Part model, mm, in its own coordinate system. A direction names the side the tool comes from. Round coordinates to 2 decimals unless told otherwise and drop trailing zeros. Write each loop counter-clockwise with the first axis right and the second up, starting at its lowest first coordinate (ties: lowest second). Pieces come first, ordered by that corner, then holes. Notation, with made-up numbers: M 31.5,62 L 67.5,62 A27 ccw 67.5,78 Z; hole C -4,42 d4. An arc over 180 degrees is marked long. Answer as a JSON object with one key per item and string values. Group by question number.
1. Band-saw the part on A-A, the plane x = 3.75. Write the cut outline in (y, z), plus the area to 3 significant figures.
2. Drill centre lines: line 1 (Z direction, x = -0.5, y = 0); line 2 (Y direction, x = 6.75, z = 6.5); line 3 (Y direction, x = 6.75, z = 0). Where is each one in solid material? Low to high. Write a range as from..to.
3. Drop flat-ended pins along their axis: pin 1 (1.5 mm diameter, centred on x = 3, z = 14.5, fed in from -Y); pin 2 (10 mm diameter, centred on y = 12.5, z = 12.5, fed in from +X); pin 3 (0.6 mm diameter, centred on y = 4, z = 4, fed in from +X). Give the stop position or say it passes through.
4. Band-saw the part on B-B, the plane y = 0. Count the separate pieces of the cut face and the enclosed holes in it, plus the area to 3 significant figures.
5. Band-saw the part on C-C, the plane x = 10. Write the cut outline in (y, z), plus the area to 3 significant figures.
6. Band-saw the part on D-D, the plane x = -0.75. Write the cut outline in (y, z).
7. Two-plate mould, pull along Z, no slides. Class faces 1 (the face through (-2.63, 13.926, 4.385)), 2 (the face through (4.105, 17.717, 5.579)), 3 (the face through (18.591, -4, 4)): +Z half, -Z half, draft (parallel to the pull), parting line (faces both ways), or undercut.
8. Which spindle directions (+Z, -Z, +X, -X, +Y, -Y) get a long thin tool onto all of the face, cutting with end or side? Do faces 4 (the face through (18.591, 0, -5)), 5 (the face through (18.084, 4.605, 3.225)), 6 (the face through (18.591, -5, 0)), 7 (the face through (18.591, 5, 0)). Say none if no direction does.
from build123d import *

# Parameters (mm, degrees)
SKETCH2_R           = 1.35
CUT_EXTRUDE1_DEPTH  = 10
SKETCH3_R           = 3.977137015
SKETCH3_R_2         = 1
BOSS_EXTRUDE1_DEPTH = 2
FILLET1_R           = 1
SKETCH4_R           = 1
CUT_EXTRUDE2_DEPTH  = 1


with BuildPart() as part:
    # Sketch1 → Revolve1 (revolve)
    with BuildSketch(Plane.XY):
        Polygon((-9.308622786, 16.6), (3.091377214, 16.6), (3.091377214, 18.57463979), (5.091377214, 18.57463979), (5.091377214, 18.07463979), (4.591377214, 18.07463979), (4.591377214, 17.07463979), (7.591377214, 14.07463979), (7.591377214, 6.75), (17.591377214, 6.75), (17.591377214, 0), (6.591377214, 0), (5.591377214, 0), (5.591377214, 13.246212665), (4.237589879, 14.6), (-9.308622786, 14.6), align=None)
    revolve(axis=Axis((-25, 0, 0), (1, 0, 0)))

    # Sketch2 → Cut-Extrude1 (cut)
    with BuildSketch(Plane.ZY.offset(-5.591377214)):
        with Locations((0, 9.5)):
            Circle(SKETCH2_R)
        with Locations((6.717514421, 6.717514421)):
            Circle(SKETCH2_R)
        with Locations((9.5, 0)):
            Circle(SKETCH2_R)
        with Locations((6.717514421, -6.717514421)):
            Circle(SKETCH2_R)
        with Locations((0, -9.5)):
            Circle(SKETCH2_R)
        with Locations((-6.717514421, -6.717514421)):
            Circle(SKETCH2_R)
        with Locations((-9.5, 0)):
            Circle(SKETCH2_R)
        with Locations((-6.717514421, 6.717514421)):
            Circle(SKETCH2_R)
    extrude(amount=-CUT_EXTRUDE1_DEPTH, mode=Mode.SUBTRACT)

    # Sketch3 → Boss-Extrude1 (add)
    with BuildSketch(Plane(origin=(17.591377214, 0, 0), x_dir=(0, 0, -1), z_dir=(1, 0, 0))):
        Circle(SKETCH3_R)
        with Locations((0, 5.320667936)):
            Circle(SKETCH3_R_2)
        with Locations((3.762280378, 3.762280378)):
            Circle(SKETCH3_R_2)
        with Locations((5.320667936, 0)):
            Circle(SKETCH3_R_2)
        with Locations((3.762280378, -3.762280378)):
            Circle(SKETCH3_R_2)
        with Locations((0, -5.320667936)):
            Circle(SKETCH3_R_2)
        with Locations((-3.762280378, -3.762280378)):
            Circle(SKETCH3_R_2)
        with Locations((-5.320667936, 0)):
            Circle(SKETCH3_R_2)
        with Locations((-3.762280378, 3.762280378)):
            Circle(SKETCH3_R_2)
    extrude(amount=BOSS_EXTRUDE1_DEPTH)

    # Fillet1
    fillet1_edges = [part.edges().sort_by_distance(p)[0] for p in [
        (19.591377214, 0, 3.977137015),
    ]]
    fillet(fillet1_edges, radius=FILLET1_R)

    # Sketch4 → Cut-Extrude2 (cut)
    with BuildSketch(Plane(origin=(19.591377214, 0, 0), x_dir=(0, 0, -1), z_dir=(1, 0, 0))):
        with Locations((0, 5.320667936)):
            Circle(SKETCH4_R)
        with Locations((3.762280378, 3.762280378)):
            Circle(SKETCH4_R)
        with Locations((5.320667936, 0)):
            Circle(SKETCH4_R)
        with Locations((3.762280378, -3.762280378)):
            Circle(SKETCH4_R)
        with Locations((0, -5.320667936)):
            Circle(SKETCH4_R)
        with Locations((-3.762280378, -3.762280378)):
            Circle(SKETCH4_R)
        with Locations((-5.320667936, 0)):
            Circle(SKETCH4_R)
        with Locations((-3.762280378, 3.762280378)):
            Circle(SKETCH4_R)
    extrude(amount=-CUT_EXTRUDE2_DEPTH, mode=Mode.SUBTRACT)


solid = part.part
Worked answers:
{
 "1": {"outline": "C 0,0 d37.15; hole C 0,0 d29.2", "area": "414 mm^2"},
 "2": {"line 1": "z = -16.6..-14.6, 14.6..16.6", "line 2": "y = -13.43..-8.05, -5.39..5.39, 8.05..13.43", "line 3": "y = -14.92..-10.85, -8.15..8.15, 10.85..14.92"},
 "3": {"pin 1": "stops at y = -12.48", "pin 2": "stops at x = 7.59", "pin 3": "stops at x = 18.59"},
 "4": {"separate pieces": "3", "enclosed holes": "0", "area": "272 mm^2"},
 "5": {"outline": "C 0,0 d13.5", "area": "143 mm^2"},
 "6": {"outline": "C 0,0 d33.2; hole C 0,0 d29.2"},
 "7": {"face 1": "undercut", "face 2": "parting line", "face 3": "draft"},
 "8": {"face 4": "-Z, +X, +Y, -Y", "face 5": "+X", "face 6": "+Z, -Z, +X, -Y", "face 7": "+Z, -Z, +X, +Y"}
}
